Source: CAD feature listing. Evaluate the final solid. Frame: model axes, mm. A direction names the side the tool comes from. Coordinates: 2 decimals unless noted, no trailing zeros. Write each loop counter-clockwise with the first axis right and the second up, starting at its lowest first coordinate (ties: lowest second). Pieces come first, ordered by that corner, then holes. Notation, with made-up numbers: M 41.5,3 L 80.5,3 A21 cw 80.5,16 Z; hole C -19,-24 d3. An arc over 180 degrees is marked long. One line per item, written item: value. Start each with the question number.
Item 1: Mould query, pull axis Y, two halves, no side actions, for faces 5 (the flat face through (39.87, 0.07, 23.32)), 6 (the cylindrical face through (-12.5, -0.93, -38.22)), 7 (the flat face through (-1, 5, -3)). Classes: released by +Y, released by -Y, zero draft, split by the parting line, or undercut.
Item 2: Ray query, L1, parallel to X at y = 1.25, z = -15; L2, parallel to X at y = 3, z = 16; L3, parallel to Z at x = 20, y = -3.85. Return the intervals inside material, ascending. Write a range as from..to.
Item 3: Pin query (flat end, axial travel): P1, Ø5.5, axis at x = -20, z = -15, coming from the -Y side; P2, Ø1.2, axis at x = -11.5, y = -1.5, coming from the -Z side; P3, Ø2.5, axis at x = -20, z = 15, coming from the +Y side; P4, Ø1.2, axis at x = -19, z = -16, coming from the +Y side. Return the tip coordinate at first contact, or that it passes through.
Item 4: Cut plane D-D, the plane z = -2. Output: boundary loops of the cut face in (x, y), then the cut area to 3 significant figures.
Item 5: Cut plane A-A, the plane y = 3.5. Output: boundary loops of the cut face in (x, z).
Item 6: Cut plane B-B, the plane x = 11. Output: boundary loops of the cut face in (y, z).
Item 7: Set-up query: faces 1 (the flat face through (0, 0, 40.415)), 2 (the cylindrical face through (9.5, -0.93, -38.22)), 3 (the cylindrical face through (21.4, 2, 13.5)), 4 (the flat face through (-25.85, -1.02, 27.6)). Return all of +Z, -Z, +X, -X, +Y, -Y with unobstructed straight access to the full face (end or side cutting, diameter ignored); none if empty.
Item 8: Cut plane C-C, the plane z = -15. Output: boundary loops of the cut face in (x, y), then the cut area to 3 significant figures.
```python
from build123d import *

# Parameters (mm, degrees)
BOSS_EXTRUDE1_DEPTH     = 5
CHAMFER1_SIZE           = 40
SKETCH4_R               = 1.5
CUT_EXTRUDE1_DEPTH      = 10
SKETCH10_R              = 2.05
CUT_EXTRUDE3_DEPTH      = 6
CRVPATTERN1_START       = -46.188021535
CRVPATTERN1_OUTLINE_R   = 2.05
CRVPATTERN1_DEPTH       = 6
CRVPATTERN1_START_2     = -40.188021535
CRVPATTERN1_2_OUTLINE_R = 1.5
CRVPATTERN1_2_DEPTH     = 4
CRVPATTERN1_3_OUTLINE_R = 2.05
CRVPATTERN1_3_DEPTH     = 6
CRVPATTERN1_4_OUTLINE_R = 1.5
CRVPATTERN1_4_DEPTH     = 4
F_3_0MM_DOWEL_HOLE1_D   = 3
FILLET1_R               = 3
SKETCH9_R               = 2.05
CUT_EXTRUDE2_DEPTH      = 6


# Read off the part's stored shape, not the designer's step: CrvPattern1
with BuildPart() as part:
    # Sketch2 → Boss-Extrude1 (new, symmetric)
    with BuildSketch(Plane(origin=(0, 0, 0), x_dir=(1, 0, 0), z_dir=(0, 1, 0))):
        Polygon((70, -40.414518843), (0, 80.829037687), (-70, -40.414518843), align=None)
    extrude(amount=BOSS_EXTRUDE1_DEPTH, both=True)

    # Chamfer1
    chamfer1_edges = [part.edges().sort_by_distance(p)[0] for p in [
        (-70, 0, 40.414518843),
        (0, 0, -80.829037687),
        (70, 0, 40.414518843),
    ]]
    chamfer(chamfer1_edges, length=CHAMFER1_SIZE)

    # Sketch4 → Cut-Extrude1 (cut)
    with BuildSketch(Plane(origin=(40, 0, 23.094010768), x_dir=(0.5000000000000004, 0, -0.8660254037844384), z_dir=(0.8660254037844384, 0, 0.5000000000000004))):
        with Locations((-11, -1)):
            Circle(SKETCH4_R)
        with Locations((11, -1)):
            Circle(SKETCH4_R)
    extrude(amount=-CUT_EXTRUDE1_DEPTH, mode=Mode.SUBTRACT)

    # Sketch10 → Cut-Extrude3 (cut)
    with BuildSketch(Plane(origin=(40, 0, 23.094010768), x_dir=(0.4999999999999997, 0, -0.8660254037844388), z_dir=(0.8660254037844389, 0, 0.49999999999999983))):
        with Locations((-11, -1)):
            Circle(SKETCH10_R)
        with Locations((11, -1)):
            Circle(SKETCH10_R)
    extrude(amount=-CUT_EXTRUDE3_DEPTH, mode=Mode.SUBTRACT)

    # CrvPattern1 outline → CrvPattern1 (cut)
    with BuildSketch(Plane.XY.offset(CRVPATTERN1_START)):
        with Locations((11, -1)):
            Circle(CRVPATTERN1_OUTLINE_R)
        with Locations((-11, -1)):
            Circle(CRVPATTERN1_OUTLINE_R)
    extrude(amount=CRVPATTERN1_DEPTH, mode=Mode.SUBTRACT)

    # CrvPattern1 2 outline → CrvPattern1 2 (cut)
    with BuildSketch(Plane.XY.offset(CRVPATTERN1_START_2)):
        with Locations((11, -1)):
            Circle(CRVPATTERN1_2_OUTLINE_R)
        with Locations((-11, -1)):
            Circle(CRVPATTERN1_2_OUTLINE_R)
    extrude(amount=CRVPATTERN1_2_DEPTH, mode=Mode.SUBTRACT)

    # CrvPattern1 3 outline → CrvPattern1 3 (cut)
    with BuildSketch(Plane(origin=(0, 0, 0), x_dir=(0.500000000000013, 0, 0.8660254037844313), z_dir=(0.8660254037844312, 0, -0.5000000000000131)).offset(CRVPATTERN1_START)):
        with Locations((-11, 1)):
            Circle(CRVPATTERN1_3_OUTLINE_R)
        with Locations((11, 1)):
            Circle(CRVPATTERN1_3_OUTLINE_R)
    extrude(amount=CRVPATTERN1_3_DEPTH, mode=Mode.SUBTRACT)

    # CrvPattern1 4 outline → CrvPattern1 4 (cut)
    with BuildSketch(Plane(origin=(0, 0, 0), x_dir=(0.500000000000013, 0, 0.8660254037844313), z_dir=(0.8660254037844312, 0, -0.5000000000000131)).offset(CRVPATTERN1_START_2)):
        with Locations((-11, 1)):
            Circle(CRVPATTERN1_4_OUTLINE_R)
        with Locations((11, 1)):
            Circle(CRVPATTERN1_4_OUTLINE_R)
    extrude(amount=CRVPATTERN1_4_DEPTH, mode=Mode.SUBTRACT)

    # Ø3.0mm Dowel Hole1 (through all)
    with Locations(Plane(origin=(0, 5, 0), x_dir=(1, 0, 0), z_dir=(0, 1, 0))):
        with Locations((-20, 15), (20, 15), (20, -15), (-20, -15)):
            Hole(F_3_0MM_DOWEL_HOLE1_D / 2)

    # Fillet1
    fillet1_edges = [part.edges().sort_by_distance(p)[0] for p in [
        (20, 0, -46.188021535),
        (50, 0, 5.773502692),
        (-30, 0, 40.414518843),
        (30, 0, 40.414518843),
        (-50, 0, 5.773502692),
        (-20, 0, -46.188021535),
    ]]
    fillet(fillet1_edges, radius=FILLET1_R)

    # Sketch9 → Cut-Extrude2 (cut)
    with BuildSketch(Plane(origin=(0, 5, 0), x_dir=(1, 0, 0), z_dir=(0, 1, 0))):
        with Locations(Location((-20, 15, 0), (0, 0, 270))):
            Circle(SKETCH9_R)
        with Locations(Location((20, 15, 0), (0, 0, 270))):
            Circle(SKETCH9_R)
        with Locations(Location((20, -15, 0), (0, 0, 270))):
            Circle(SKETCH9_R)
        with Locations(Location((-20, -15, 0), (0, 0, 270))):
            Circle(SKETCH9_R)
    extrude(amount=-CUT_EXTRUDE2_DEPTH, mode=Mode.SUBTRACT)


solid = part.part
```
From the geometry:
1. face 5: zero draft
1. face 6: undercut
1. face 7: released by +Y
2. L1: x = -38.01..-22.05, -17.95..17.95, 22.05..38.01
2. L2: x = -44.1..-21.79, -18.21..18.21, 21.79..44.1
2. L3: z = -45.64..-16.5, -13.5..13.5, 16.5..40.41
3. P1: stops at y = -5
3. P2: stops at z = -36.19
3. P3: passes through
3. P4: stops at y = -1
4. outline: M -45.51,-5 L 45.51,-5 L 45.51,5 L -45.51,5 Z
4. area: 910 mm²
5. outline: M -49.13,4.27 L -20.87,-44.69 A3 ccw -18.27,-46.19 L 18.27,-46.19 A3 ccw 20.87,-44.69 L 49.13,4.27 A3 ccw 49.13,7.27 L 30.87,38.91 A3 ccw 28.27,40.41 L -28.27,40.41 A3 ccw -30.87,38.91 L -49.13,7.27 A3 ccw Z; hole C -20,-15 d4.1; hole C -20,15 d4.1; hole C 20,-15 d4.1; hole C 20,15 d4.1
6. outline: M -5,-46.19 L -3.05,-46.19 L -3.05,-40.19 L -2.5,-40.19 L -2.5,-36.19 L 0.5,-36.19 L 0.5,-40.19 L 1.05,-40.19 L 1.05,-46.19 L 5,-46.19 L 5,40.41 L -5,40.41 Z
7. face 1: +Z, +X, -X, +Y, -Y
7. face 2: -Z
7. face 3: +Y
7. face 4: none
8. outline: M -38.01,-5 L -21.5,-5 L -21.5,-1 L -22.05,-1 L -22.05,5 L -38.01,5 Z; M -18.5,-5 L 18.5,-5 L 18.5,-1 L 17.95,-1 L 17.95,5 L -17.95,5 L -17.95,-1 L -18.5,-1 Z; M 21.5,-5 L 38.01,-5 L 38.01,5 L 22.05,5 L 22.05,-1 L 21.5,-1 Z
8. area: 687 mm²
